Here's the drawing with two shaded views (mm, measured from the low corner). I have some questions. Round coordinates to 2 decimals unless told otherwise and drop trailing zeros. Order: outer loops, then holes, each group sorted by start corner. A loop starts at its lowest first (then second) coordinate and runs counter-clockwise, first axis right, second up. Notation, with made-up numbers: (-16.75, 67.5) -> (3.25, 67.5) arc R24 cw to (3.25, 103.5) -> close; hole circle Ø3 at (76.5, 59.5). An arc over 180 degrees is marked (long way). Answer in a Markdown table with one row per item.
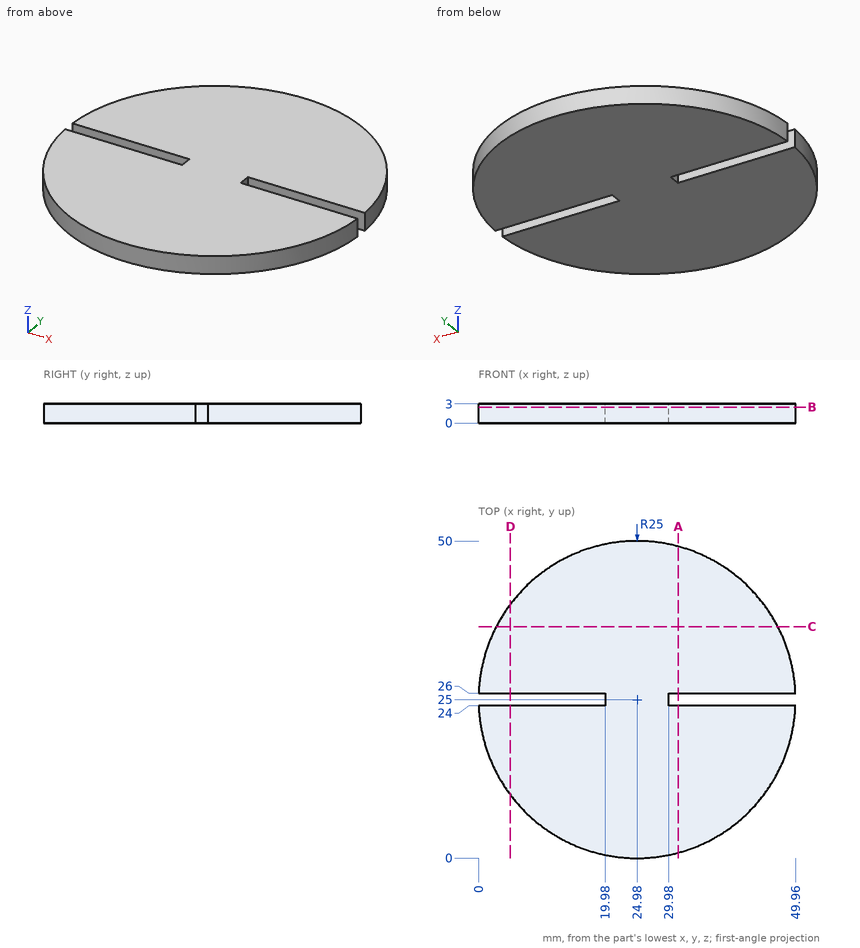
1. Suppose I cut it at D-D on x = 5. Write out the boundary of the cut face in (y, z).
Numbers:
| item | result |
|---|---|
| outline | (9.97, 0) -> (24, 0) -> (24, 3) -> (9.97, 3) -> close; (26, 0) -> (40.03, 0) -> (40.03, 3) -> (26, 3) -> close |
2. Suppose I cut it at C-C on y = 36.5. Write out the boundary of the cut face in (x, z).
Numbers:
| item | result |
|---|---|
| outline | (2.78, 0) -> (47.18, 0) -> (47.18, 3) -> (2.78, 3) -> close |
3. Suppose I cut it at B-B on z = 2.5. Write out the boundary of the cut face in (x, y), then the cut area to 3 significant figures.
Numbers:
| item | result |
|---|---|
| outline | (0, 24) arc R25 ccw to (49.96, 24) -> (29.98, 24) -> (29.98, 26) -> (49.96, 26) arc R25 ccw to (0, 26) -> (19.98, 26) -> (19.98, 24) -> close |
| area | 1,880 mm2 |
4. Please list where these lines run through material, in increasing order: line 1 along Y through (x, z) = (40, 0.25) (3 decimals); line 2 along Y through (x, z) = (17.5, 0.85); line 3 along X through (y, z) = (2, 0.9).
Numbers:
| item | result |
|---|---|
| line 1 | y = 5.015 to 24, 26 to 44.985 |
| line 2 | y = 1.15 to 24, 26 to 48.85 |
| line 3 | x = 15.18 to 34.78 |
5. Suppose I cut it at A-A on x = 31.5. Write out the boundary of the cut face in (y, z).
Numbers:
| item | result |
|---|---|
| outline | (0.87, 0) -> (24, 0) -> (24, 3) -> (0.87, 3) -> close; (26, 0) -> (49.13, 0) -> (49.13, 3) -> (26, 3) -> close |
6. For pin 1 Ø1.5 at (x, z) = (11.5, 1.5) entering from +Y; pin 2 Ø1.5 at (x, z) = (37, 1) entering from +Y; pin 3 Ø0.9 at (x, z) = (12, 1.5) entering from -Y, each with a flat end and sliding along its axis, tell me the tip position at first contact or that it passes through.
Numbers:
| item | result |
|---|---|
| pin 1 | stops at y = 46.52 |
| pin 2 | stops at y = 47.32 |
| pin 3 | stops at y = 3.37 |
